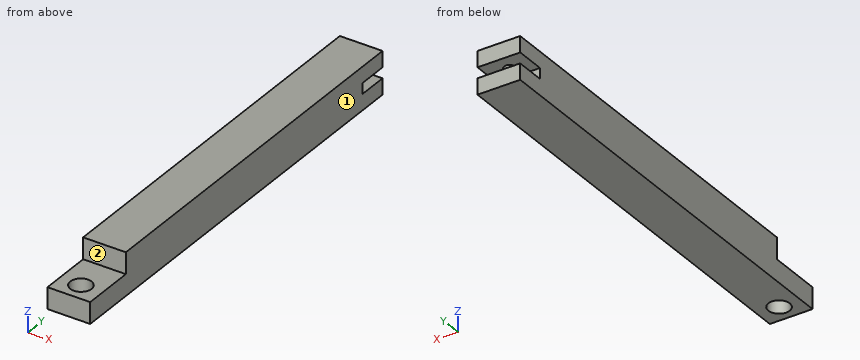
```python
from build123d import *

# Parameters (mm, degrees)
F1_DEPTH = 25.4
F2_W     = 31.75
F2_H     = 12.7
F3_DEPTH = 25.4
F4_R     = 3.175
F5_DEPTH = 25.4
F6_R     = 6.35
F7_DEPTH = 25.4


with BuildPart() as f1:
    # F0 (on Right) → F1 (new body)
    with BuildSketch(Plane.YZ):
        Polygon((0, 25.4), (0, 0), (260.35, 0), (260.35, 9.525), (242.712691, 9.525), (242.712691, 15.875), (260.35, 15.875), (260.35, 25.4), align=None)
    extrude(amount=F1_DEPTH)

    # F2 (on face) → F3 (cut)
    with BuildSketch(Plane.YZ.offset(25.4)):
        with Locations((15.875, 19.05)):
            Rectangle(F2_W, F2_H)
    extrude(amount=-F3_DEPTH, mode=Mode.SUBTRACT)

    # F4 (on face) → F5 (join)
    with BuildSketch(Plane(origin=(0, 0, 0), x_dir=(1, 0, 0), z_dir=(0, 0, -1))):
        with Locations((12.7, -250.825)):
            Circle(F4_R)
    extrude(amount=-F5_DEPTH)

    # F6 (on face) → F7 (cut)
    with BuildSketch(Plane.XY.offset(12.7)):
        with Locations((12.7, 10.795)):
            Circle(F6_R)
    extrude(amount=-F7_DEPTH, mode=Mode.SUBTRACT)


solid = f1.part
```
Work out the finished part from the listing and answer in its coordinate system (mm). Face numbers are marked on the shaded views. A direction names the side the tool comes from. Coordinates: 2 decimals unless noted, no trailing zeros. Loops run counter-clockwise (first coordinate to the right, second up) from the corner with the lowest first, then second, coordinate; pieces in that order, holes last.
1) Section B-B (x = 23.25) is taken. Give the vertices of the cut face in (y, z) (3 decimals), plus the area to 3 significant figures.
Results:
outline: (0, 0) - (260.35, 0) - (260.35, 9.525) - (242.713, 9.525) - (242.713, 15.875) - (260.35, 15.875) - (260.35, 25.4) - (31.75, 25.4) - (31.75, 12.7) - (0, 12.7) - close
area: 6,100 mm2
2) For the marked faces 1 and 2, determine the directions among +Z, -Z, +X, -X, +Y, -Y from which every point of the face is accessible in a straight line to the end or side of a thin tool.
Results:
face 1: +Z, -Z, +X, +Y, -Y
face 2: +Z, +X, -X, -Y
3) Consider probe 1 along Y at (x, z) = (12.7, 7.5) (3 decimals); probe 2 along Z at (x, y) = (10.5, 244) (3 decimals); probe 3 along Y at (x, z) = (22.75, 20.75). Determine where each line is inside the solid, lowest interval first.
Results:
probe 1: y = 0 to 4.445, 17.145 to 260.35
probe 2: z = 0 to 9.525, 15.875 to 25.4
probe 3: y = 31.75 to 260.35
4) Section A-A (x = 12.7) is taken. Give the vertices of the cut face in (y, z) (3 decimals).
Results:
outline: (0, 0) - (4.445, 0) - (4.445, 12.7) - (0, 12.7) - close; (17.145, 0) - (260.35, 0) - (260.35, 9.525) - (254, 9.525) - (254, 15.875) - (260.35, 15.875) - (260.35, 25.4) - (31.75, 25.4) - (31.75, 12.7) - (17.145, 12.7) - close; hole (242.713, 9.525) - (247.65, 9.525) - (247.65, 15.875) - (242.713, 15.875) - close
5) Flat-ended cylindrical pins translate along their axes: pin 1 (4 mm diameter, centred on x = 11.5, z = 19.5, fed in from -Y); pin 2 (14.5 mm diameter, centred on x = 12.7, y = 10.795, fed in from +Z); pin 3 (1.9 mm diameter, centred on x = 10.5, z = 14, fed in from +Y). Find the tip coordinate at first contact, or state that the pin passes through.
Results:
pin 1: stops at y = 31.75
pin 2: stops at z = 12.7
pin 3: stops at y = 253.74
6) Section C-C (z = 19.25) is taken. Give the vertices of the cut face in (x, y), plus the area to 3 significant figures.
Results:
outline: (0, 31.75) - (25.4, 31.75) - (25.4, 260.35) - (0, 260.35) - close
area: 5,810 mm2
7) Section D-D (y = 28.5) is taken. Give the vertices of the cut face in (x, z), plus the area to 3 significant figures.
Results:
outline: (0, 0) - (25.4, 0) - (25.4, 12.7) - (0, 12.7) - close
area: 323 mm2
